Geometry check sheet. Reference: the model listing, model coordinates, mm. Face numbers are marked on the shaded views. A direction names the side the tool comes from. Round coordinates to 2 decimals unless told otherwise and drop trailing zeros. Loops run counter-clockwise (first coordinate to the right, second up) from the corner with the lowest first, then second, coordinate; pieces in that order, holes last.
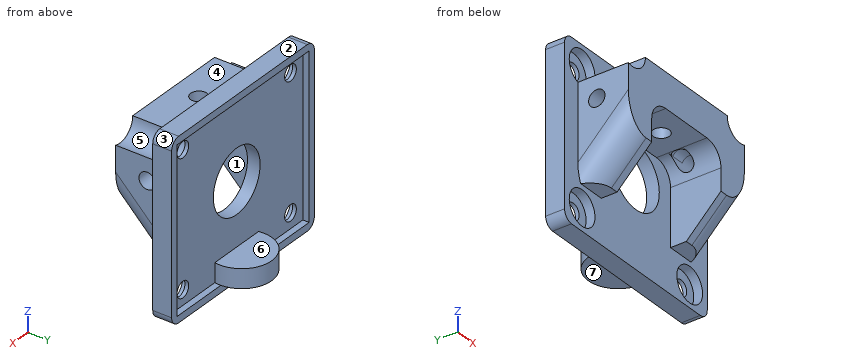
```python
from build123d import *

# Parameters (mm, degrees)
SKETCH_1_W           = 30.5
SKETCH_1_H           = 28
EXTRUDE_1_DEPTH      = 1.6
SKETCH_2_W           = 28.25
SKETCH_2_H           = 25.75
CUT_EXTRUDE_1_DEPTH  = 1
EXTRUDE_2_DEPTH      = 3
CUT_EXTRUDE_2_REACH  = 43.774
SKETCH_5_R           = 1.25
CUT_EXTRUDE_3_REACH  = 43.774
SKETCH_6_R           = 5
SKETCH_7_W           = 30.5
SKETCH_7_H           = 28
SKETCH_7_R           = 2.75
SKETCH_7_R_2         = 5
EXTRUDE_3_DEPTH      = 1.4
SKETCH_8_W           = 5
SKETCH_8_H           = 14
EXTRUDE_4_DEPTH      = 10
CUT_EXTRUDE_4_DEPTH  = 41.969287277
SKETCH_10_W          = 24.8
SKETCH_10_H          = 10
EXTRUDE_5_DEPTH      = 3.5
SKETCH_11_R          = 2.75
CUT_EXTRUDE_5_DEPTH  = 43.944266206
SKETCH_12_R          = 1.3
CUT_EXTRUDE_6_DEPTH  = 41.969287277
CUT_EXTRUDE_7_REACH  = 42.749
SKETCH_13_R          = 1.3
CUT_EXTRUDE_8_REACH  = 42.969
SKETCH_14_W          = 12
SKETCH_14_H          = 2
SKETCH_15_W          = 14.8
SKETCH_15_H          = 8
SKETCH_15_R          = 1.3
EXTRUDE_6_DEPTH      = 2
FILLET_1_R           = 3.8
FILLET_2_R           = 1.5
FILLET_3_R           = 3
CUT_EXTRUDE_START    = -3
CUT_EXTRUDE_9_DEPTH  = 3
CUT_EXTRUDE_10_DEPTH = 3
FILLET_4_R           = 1


with BuildPart() as part:
    # 草图1 → 凸台-拉伸1 (new body)
    with BuildSketch(Plane(origin=(0, 0, 0), x_dir=(1, 0, 0), z_dir=(0, 1, 0))):
        with Locations((15.25, 14)):
            Rectangle(SKETCH_1_W, SKETCH_1_H)
    extrude(amount=EXTRUDE_1_DEPTH)

    # 草图2 → 切除-拉伸1 (cut)
    with BuildSketch(Plane(origin=(0, 1.6, 0), x_dir=(1, 0, 0), z_dir=(0, 1, 0))):
        with Locations((15.25, 14)):
            Rectangle(SKETCH_2_W, SKETCH_2_H)
    extrude(amount=-CUT_EXTRUDE_1_DEPTH, mode=Mode.SUBTRACT)

    # 草图3 → 凸台-拉伸2 (add)
    with BuildSketch(Plane(origin=(57.75, 0, -26.875), x_dir=(1, 0, 0), z_dir=(0, 0, 1))):
        with BuildLine():
            Line((-47.182146943, 0.6), (-37.817853057, 0.6))
            ThreePointArc((-37.817853057, 0.6), (-42.5, 6.15), (-47.182146943, 0.6))
        make_face()
    extrude(amount=EXTRUDE_2_DEPTH)

    # 草图5 → 切除-拉伸2 (cut, up to next)
    with BuildSketch(Plane(origin=(0, 0.6, 0), x_dir=(1, 0, 0), z_dir=(0, 1, 0)), mode=Mode.PRIVATE) as cut_extrude_2_sk1:
        with Locations(Location((3.75, 24.5, 0), (0, 0, 270))):
            Circle(SKETCH_5_R)
    cut_extrude_2_tool1 = extrude(cut_extrude_2_sk1.sketch, amount=-CUT_EXTRUDE_2_REACH, mode=Mode.PRIVATE) & part.part
    # 草图5 → 切除-拉伸2 (cut, up to next)
    with BuildSketch(Plane(origin=(0, 0.6, 0), x_dir=(1, 0, 0), z_dir=(0, 1, 0)), mode=Mode.PRIVATE) as cut_extrude_2_sk2:
        with Locations(Location((26.75, 24.5, 0), (0, 0, 270))):
            Circle(SKETCH_5_R)
    cut_extrude_2_tool2 = extrude(cut_extrude_2_sk2.sketch, amount=-CUT_EXTRUDE_2_REACH, mode=Mode.PRIVATE) & part.part
    # 草图5 → 切除-拉伸2 (cut, up to next)
    with BuildSketch(Plane(origin=(0, 0.6, 0), x_dir=(1, 0, 0), z_dir=(0, 1, 0)), mode=Mode.PRIVATE) as cut_extrude_2_sk3:
        with Locations(Location((3.75, 3.5, 0), (0, 0, 270))):
            Circle(SKETCH_5_R)
    cut_extrude_2_tool3 = extrude(cut_extrude_2_sk3.sketch, amount=-CUT_EXTRUDE_2_REACH, mode=Mode.PRIVATE) & part.part
    # 草图5 → 切除-拉伸2 (cut, up to next)
    with BuildSketch(Plane(origin=(0, 0.6, 0), x_dir=(1, 0, 0), z_dir=(0, 1, 0)), mode=Mode.PRIVATE) as cut_extrude_2_sk4:
        with Locations(Location((26.75, 3.5, 0), (0, 0, 270))):
            Circle(SKETCH_5_R)
    cut_extrude_2_tool4 = extrude(cut_extrude_2_sk4.sketch, amount=-CUT_EXTRUDE_2_REACH, mode=Mode.PRIVATE) & part.part
    add(cut_extrude_2_tool1.solids().sort_by_distance((3.75, 0.6, -24.5))[0], mode=Mode.SUBTRACT)
    add(cut_extrude_2_tool2.solids().sort_by_distance((26.75, 0.6, -24.5))[0], mode=Mode.SUBTRACT)
    add(cut_extrude_2_tool3.solids().sort_by_distance((3.75, 0.6, -3.5))[0], mode=Mode.SUBTRACT)
    add(cut_extrude_2_tool4.solids().sort_by_distance((26.75, 0.6, -3.5))[0], mode=Mode.SUBTRACT)

    # 草图6 → 切除-拉伸3 (cut, up to next)
    with BuildSketch(Plane(origin=(0, 0.6, 0), x_dir=(1, 0, 0), z_dir=(0, 1, 0)), mode=Mode.PRIVATE) as cut_extrude_3_sk1:
        with Locations(Location((15.25, 14, 0), (0, 0, 270))):
            Circle(SKETCH_6_R)
    cut_extrude_3_tool1 = extrude(cut_extrude_3_sk1.sketch, amount=-CUT_EXTRUDE_3_REACH, mode=Mode.PRIVATE) & part.part
    add(cut_extrude_3_tool1.solids().sort_by_distance((15.25, 0.6, -14))[0], mode=Mode.SUBTRACT)

    # 草图7 → 凸台-拉伸3 (add)
    with BuildSketch(Plane.XZ):
        with Locations((15.25, -14)):
            Rectangle(SKETCH_7_W, SKETCH_7_H)
        with Locations(Location((3.75, -3.5, 0), (0, 0, 270))):
            Circle(SKETCH_7_R, mode=Mode.SUBTRACT)
        with Locations(Location((26.75, -3.5, 0), (0, 0, 270))):
            Circle(SKETCH_7_R, mode=Mode.SUBTRACT)
        with Locations(Location((3.75, -24.5, 0), (0, 0, 270))):
            Circle(SKETCH_7_R, mode=Mode.SUBTRACT)
        with Locations(Location((26.75, -24.5, 0), (0, 0, 270))):
            Circle(SKETCH_7_R, mode=Mode.SUBTRACT)
        with Locations(Location((15.25, -14, 0), (0, 0, 90))):
            Circle(SKETCH_7_R_2, mode=Mode.SUBTRACT)
    extrude(amount=EXTRUDE_3_DEPTH)

    # 草图8 → 凸台-拉伸4 (add)
    with BuildSketch(Plane.XZ.offset(1.4)):
        with Locations((25.15, -14)):
            Rectangle(SKETCH_8_W, SKETCH_8_H)
        with Locations((5.35, -14)):
            Rectangle(SKETCH_8_W, SKETCH_8_H)
    extrude(amount=EXTRUDE_4_DEPTH)

    # 草图9 → 切除-拉伸4 (cut, through all)
    with BuildSketch(Plane.ZY.offset(-2.85)):
        Polygon((-21, -3.9), (-13.5, -11.4), (-21, -11.4), align=None)
    extrude(amount=-CUT_EXTRUDE_4_DEPTH, mode=Mode.SUBTRACT)

    # 草图10 → 凸台-拉伸5 (add)
    with BuildSketch(Plane.XY.offset(-7)):
        with Locations((15.25, -6.4)):
            Rectangle(SKETCH_10_W, SKETCH_10_H)
    extrude(amount=EXTRUDE_5_DEPTH)

    # 草图11 → 切除-拉伸5 (cut, through all)
    with BuildSketch(Plane.XZ):
        with Locations(Location((26.75, -3.5, 0), (0, 0, 180))):
            Circle(SKETCH_11_R)
        with Locations((3.75, -3.5)):
            Circle(SKETCH_11_R)
    extrude(amount=CUT_EXTRUDE_5_DEPTH, mode=Mode.SUBTRACT)

    # 草图12 → 切除-拉伸6 (cut, through all)
    with BuildSketch(Plane.ZY.offset(-2.85)):
        with Locations((-9.598557292, -4.4)):
            Circle(SKETCH_12_R)
    extrude(amount=-CUT_EXTRUDE_6_DEPTH, mode=Mode.SUBTRACT)

    # 草图13 → 切除-拉伸7 (cut, up to next)
    with BuildSketch(Plane.XY.offset(-3.5), mode=Mode.PRIVATE) as cut_extrude_7_sk1:
        with Locations((15.25, -5.4)):
            Circle(SKETCH_13_R)
    cut_extrude_7_tool1 = extrude(cut_extrude_7_sk1.sketch, amount=-CUT_EXTRUDE_7_REACH, mode=Mode.PRIVATE) & part.part
    add(cut_extrude_7_tool1.solids().sort_by_distance((15.25, -5.4, -3.5))[0], mode=Mode.SUBTRACT)

    # 草图14 → 切除-拉伸8 (cut, up to next)
    with BuildSketch(Plane(origin=(27.65, 0, 0), x_dir=(0, 0, -1), z_dir=(1, 0, 0)), mode=Mode.PRIVATE) as cut_extrude_8_sk1:
        with Locations((9.5, -10.4)):
            Rectangle(SKETCH_14_W, SKETCH_14_H)
    cut_extrude_8_tool1 = extrude(cut_extrude_8_sk1.sketch, amount=-CUT_EXTRUDE_8_REACH, mode=Mode.PRIVATE) & part.part
    add(cut_extrude_8_tool1.solids().sort_by_distance((27.65, -10.4, -9.5))[0], mode=Mode.SUBTRACT)

    # 草图15 → 凸台-拉伸6 (add)
    with BuildSketch(Plane(origin=(0, 0, -7), x_dir=(-1, 0, 0), z_dir=(0, 0, -1))):
        with Locations((-15.25, -5.4)):
            Rectangle(SKETCH_15_W, SKETCH_15_H)
        with Locations(Location((-15.25, -5.4, 0), (0, 0, 180))):
            Circle(SKETCH_15_R, mode=Mode.SUBTRACT)
    extrude(amount=EXTRUDE_6_DEPTH)

    # 圆角1
    fillet_1_edges = [part.edges().sort_by_distance(p)[0] for p in [
        (27.65, -6.65, -18.25),
        (2.85, -6.65, -18.25),
    ]]
    fillet(fillet_1_edges, radius=FILLET_1_R)

    # 圆角2
    fillet_2_edges = [part.edges().sort_by_distance(p)[0] for p in [
        (0, 0.1, -28),
        (30.5, 0.1, -28),
        (30.5, 0.1, 0),
        (0, 0.1, 0),
    ]]
    fillet(fillet_2_edges, radius=FILLET_2_R)

    # 圆角3
    # the kernel refuses this fillet: 3 mm, written as the material it adds along each edge
    with BuildSketch(Plane(origin=(22.65, 6.1, -9), x_dir=(0, 0, -1), z_dir=(0, -1, 0))) as fillet_3_piece_1_section:
        with BuildLine():
            CenterArc((FILLET_3_R, -FILLET_3_R), FILLET_3_R, 90, 90)
            Line((0, -FILLET_3_R), (0, 0))
            Line((0, 0), (FILLET_3_R, 0))
        make_face()
    fillet_3_piece_1 = extrude(amount=16.845994295, mode=Mode.PRIVATE)
    fillet_3_piece_1 = split(fillet_3_piece_1, bisect_by=Plane(origin=(22.65, -9.4, -9), z_dir=(0, 1, 0)), keep=Keep.TOP, mode=Mode.PRIVATE)
    fillet_3_piece_1 = fillet_3_piece_1 - Plane(origin=(22.65, -4.4, -9.598557292), x_dir=(0, 0, 1), z_dir=(-1, 0, 0)) * Cylinder(1.3, 46, mode=Mode.PRIVATE)
    fillet_3_piece_1 = split(fillet_3_piece_1, bisect_by=Plane(origin=(22.65, 0.6, -9), z_dir=(0, -1, 0)), keep=Keep.TOP, mode=Mode.PRIVATE)
    add(fillet_3_piece_1)
    with BuildSketch(Plane(origin=(7.85, -10.745994295, -9), x_dir=(1, 0, 0), z_dir=(0, 1, 0))) as fillet_3_piece_2_section:
        with BuildLine():
            CenterArc((FILLET_3_R, FILLET_3_R), FILLET_3_R, 180, 90)
            Line((0, FILLET_3_R), (0, 0))
            Line((0, 0), (FILLET_3_R, 0))
        make_face()
    fillet_3_piece_2 = extrude(amount=16.845994295, mode=Mode.PRIVATE)
    fillet_3_piece_2 = split(fillet_3_piece_2, bisect_by=Plane(origin=(7.85, -9.4, -9), z_dir=(0, 1, 0)), keep=Keep.TOP, mode=Mode.PRIVATE)
    fillet_3_piece_2 = fillet_3_piece_2 - Plane(origin=(7.85, -4.4, -9.598557292), x_dir=(0, 0, 1), z_dir=(-1, 0, 0)) * Cylinder(1.3, 46, mode=Mode.PRIVATE)
    fillet_3_piece_2 = split(fillet_3_piece_2, bisect_by=Plane(origin=(7.85, 0.6, -9), z_dir=(0, -1, 0)), keep=Keep.TOP, mode=Mode.PRIVATE)
    add(fillet_3_piece_2)

    # 草图16 → 切除-拉伸9 (cut)
    with BuildSketch(Plane(origin=(22.65, 0, 0), x_dir=(0, 0, -1), z_dir=(1, 0, 0)).offset(CUT_EXTRUDE_START)):
        with BuildLine():
            Line((9, -5.554005705), (9, -3.245994295))
            ThreePointArc((9, -3.245994295), (8.298557292, -4.4), (9, -5.554005705))
        make_face()
    extrude(amount=CUT_EXTRUDE_9_DEPTH, mode=Mode.SUBTRACT)

    # 草图17 → 切除-拉伸10 (cut)
    with BuildSketch(Plane.ZY.offset(-7.85)):
        with BuildLine():
            Line((-9, -3.245994295), (-9, -5.554005705))
            ThreePointArc((-9, -5.554005705), (-8.298557292, -4.4), (-9, -3.245994295))
        make_face()
    extrude(amount=-CUT_EXTRUDE_10_DEPTH, mode=Mode.SUBTRACT)

    # 圆角4
    # the kernel refuses this fillet: 1 mm, written as the material it adds along each edge
    with BuildSketch(Plane(origin=(10.85, -4.4, -9.598557292), x_dir=(0, -0.12437985627786666, -0.9922346755441966), z_dir=(0, 0.9922346755441966, -0.12437985627786666))) as fillet_4_piece_1_section:
        with BuildLine():
            CenterArc((1.3 - FILLET_4_R, FILLET_4_R), FILLET_4_R, 270, 90)
            Line((1.3 - FILLET_4_R, 0), (1.3, 0))
            Line((1.3, 0), (1.3, FILLET_4_R))
        make_face()
    fillet_4_piece_1 = revolve(axis=Axis((10.85, -4.4, -9.598557292), (-1, 0, 0)), revolution_arc=345.710110631, mode=Mode.PRIVATE)
    fillet_4_piece_1 = split(fillet_4_piece_1, bisect_by=Plane(origin=(10.85, -4.4, -9), z_dir=(0, 0, 1)), keep=Keep.TOP, mode=Mode.PRIVATE)
    add(fillet_4_piece_1)
    with BuildSketch(Plane(origin=(19.65, -4.4, -9.598557292), x_dir=(0, 0.12437985627786262, -0.9922346755441972), z_dir=(0, -0.9922346755441972, -0.12437985627786262))) as fillet_4_piece_2_section:
        with BuildLine():
            CenterArc((1.3 - FILLET_4_R, FILLET_4_R), FILLET_4_R, 270, 90)
            Line((1.3, FILLET_4_R), (1.3, 0))
            Line((1.3, 0), (1.3 - FILLET_4_R, 0))
        make_face()
    fillet_4_piece_2 = revolve(axis=Axis((19.65, -4.4, -9.598557292), (1, 0, 0)), revolution_arc=345.710110631, mode=Mode.PRIVATE)
    fillet_4_piece_2 = split(fillet_4_piece_2, bisect_by=Plane(origin=(19.65, -4.4, -9), z_dir=(0, 0, 1)), keep=Keep.TOP, mode=Mode.PRIVATE)
    add(fillet_4_piece_2)


solid = part.part
```
1) Sectioned sample at A-A, the plane z = -24.5. Record the cut outline in (x, y) (3 decimals).
Report:
outline: (0, -1.4) - (1, -1.4) - (1, 0) - (2.5, 0) - (2.5, 0.6) - (1.125, 0.6) - (1.125, 1.6) - (0, 1.6) - close; (5, 0) - (6.5, 0) - (6.5, -1.4) - (24, -1.4) - (24, 0) - (25.5, 0) - (25.5, 0.6) - (19.932, 0.6) arc R4.75 ccw (long way) to (10.568, 0.6) - (5, 0.6) - close; (28, 0) - (29.5, 0) - (29.5, -1.4) - (30.5, -1.4) - (30.5, 1.6) - (29.375, 1.6) - (29.375, 0.6) - (28, 0.6) - close
2) Sectioned sample at D-D, the plane x = 21.5. Record the cut outline in (y, z) (3 decimals).
Report:
outline: (-9.4, -9.638) - (-5.699, -9.638) arc R1.3 cw (long way) to (-3.101, -9.638) - (-1.4, -9.638) - (-1.4, -28) - (1.6, -28) - (1.6, -26.875) - (0.6, -26.875) - (0.6, -1.125) - (1.6, -1.125) - (1.6, 0) - (-1.4, 0) - (-1.4, -3.5) - (-9.4, -3.5) - close
3) Sectioned sample at B-B, the plane y = -1. Record the cut outline in (x, z), then the cut area to 3 significant figures.
Report:
outline: (0, -26.5) arc R1.5 ccw to (1.5, -28) - (29, -28) arc R1.5 ccw to (30.5, -26.5) - (30.5, -1.5) arc R1.5 ccw to (29, 0) - (1.5, 0) arc R1.5 ccw to (0, -1.5) - close; hole circle Ø5.5 at (3.75, -24.5); hole circle Ø5.5 at (3.75, -3.5); hole circle Ø10 at (15.25, -14); hole circle Ø5.5 at (26.75, -24.5); hole circle Ø5.5 at (26.75, -3.5)
area: 678 mm2
4) Scan lines: line 1 along X through (y, z) = (0.4, -24.5); line 2 along X through (y, z) = (1, -16.5) (3 decimals); line 3 along X through (y, z) = (-0.65, -24.5). Record each from-to range of solid material in increasing order.
Report:
line 1: x = 0 to 2.5, 5 to 25.5, 28 to 30.5
line 2: x = 0 to 1.125, 29.375 to 30.5
line 3: x = 0 to 1, 6.5 to 24, 29.5 to 30.5
5) Gauge pin test, flat ends, axial feed: pin 1 (0.5 mm diameter, centred on x = 20, y = -5, fed in from -Z); pin 2 (5 mm diameter, centred on y = -8, z = -11, fed in from +X); pin 3 (3 mm diameter, centred on y = -7.5, z = -17, fed in from -X); pin 4 (2 mm diameter, centred on x = 3.75, z = -24.5, fed in from +Y). Record the tip position at first contact, or that the pin passes through.
Report:
pin 1: stops at z = -9
pin 2: stops at x = 27.65
pin 3: stops at x = 3.43
pin 4: passes through
6) Access from +Z, -Z, +X, -X, +Y, -Y to the whole of each face (thin tool, end or side, straight path). Record for the marked faces 4, 5, 6 and 7.
Report:
face 4: +Z, +X, -X, -Y
face 5: -Y
face 6: +Y
face 7: -Z, +X, -X, +Y
7) Sectioned sample at C-C, the plane x = 12. Record the cut outline in (y, z) (3 decimals), then the cut area to 3 significant figures.
Report:
outline: (-9.4, -9) - (-1.4, -9) - (-1.4, -10.2) - (0.6, -10.2) - (0.6, -1.125) - (1.6, -1.125) - (1.6, 0) - (-1.4, 0) - (-1.4, -3.5) - (-9.4, -3.5) - close; (-1.4, -28) - (1.6, -28) - (1.6, -26.875) - (4.864, -26.875) - (4.864, -23.875) - (0.6, -23.875) - (0.6, -17.8) - (-1.4, -17.8) - close
area: 99.8 mm2
8) Mould release check, pull along X, two halves, no side actions. Record for the marked faces 1, 2 and 3: +X half, -X half, draft (parallel to the pull), parting line (faces both ways), or undercut.
Report:
face 1: undercut
face 2: draft
face 3: +X half
